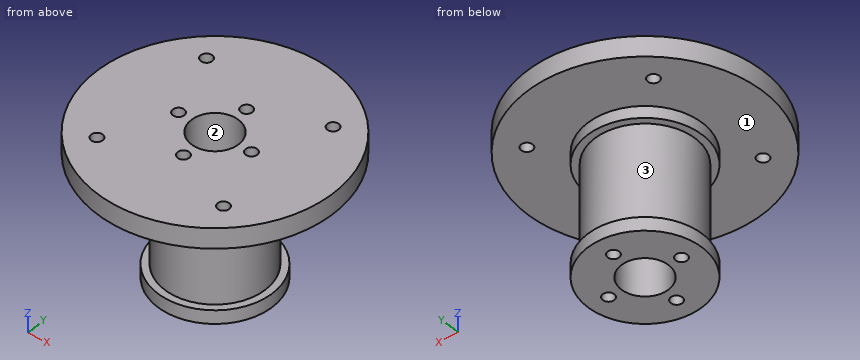
Solid Edge part; units mm, degrees
sketch "Sketch1" plane through (0, 0, 0) normal (0, 0, 1) x (1, 0, 0)
  circle A0 centre (0, 0) radius 17
  circle A1 centre (0, 0) radius 7
  circle A2 centre (11, 0) radius 1.7
  circle A3 centre (0, 11) radius 1.7
  circle A4 centre (-11, 0) radius 1.7
  circle A5 centre (0, -11) radius 1.7
extrude "Protrusion1" add sketch "Sketch1" along normal blind 4
sketch "Sketch2" plane through (0, 0, 4) normal (0, 0, 1) x (1, 0, 0)
  circle A0 centre (0, 0) radius 14.925
  circle A1 centre (0, 0) radius 7
  circle A2 centre (11, 0) radius 1.7
  circle A3 centre (0, 11) radius 1.7
  circle A4 centre (-11, 0) radius 1.7
  circle A5 centre (0, -11) radius 1.7
extrude "ExtrudedProtrusion_2" add sketch "Sketch2" along normal blind 29
sketch "Sketch3" plane through (0, 0, 33) normal (0, 0, 1) x (1, 0, 0)
  circle A0 centre (0, 0) radius 17
  circle A1 centre (0, 0) radius 7
  circle A2 centre (11, 0) radius 1.7
  circle A3 centre (0, 11) radius 1.7
  circle A4 centre (-11, 0) radius 1.7
  circle A5 centre (0, -11) radius 1.7
extrude "ExtrudedProtrusion_3" add sketch "Sketch3" along normal blind 3.5
sketch "Sketch4" plane through (0, 0, 36.5) normal (0, 0, 1) x (1, 0, 0)
  circle A0 centre (0, 0) radius 35
  circle A1 centre (0, 0) radius 7
  circle A2 centre (11, 0) radius 1.7
  circle A3 centre (0, 11) radius 1.7
  circle A4 centre (-11, 0) radius 1.7
  circle A5 centre (0, -11) radius 1.7
  circle A6 centre (19.0919, 19.0919) radius 1.7
  circle A7 centre (-19.0919, 19.0919) radius 1.7
  circle A8 centre (-19.0919, -19.0919) radius 1.7
  circle A9 centre (19.0919, -19.0919) radius 1.7
extrude "ExtrudedProtrusion_4" add sketch "Sketch4" along normal blind 6
Verification items for the finished model (mm, model axes). Face numbers are marked on the shaded views. Round coordinates to 2 decimals unless told otherwise and drop trailing zeros. Order: outer loops, then holes, each group sorted by start corner. A loop starts at its lowest first (then second) coordinate and runs counter-clockwise, first axis right, second up.
1) Depth check by flat-ended pin: pin 1 (5.5 mm diameter, centred on x = 11, y = 0, fed in from -Z); pin 2 (8 mm diameter, centred on y = -17, z = 37, fed in from -X); pin 3 (1.5 mm diameter, centred on x = 8, z = 12.5, fed in from +Y); pin 4 (4 mm diameter, centred on y = -13, z = 11, fed in from -X). Enter the tip coordinate at first touch or a pass-through.
Geometry says:
pin 1: stops at z = 0
pin 2: stops at x = -32.5
pin 3: stops at y = 13.05
pin 4: stops at x = -10.09
2) Draft check along X on the marked faces 1, 2 and 3. Enter one of: +X half, -X half, draft (parallel to the pull), parting line (faces both ways), or undercut.
Geometry says:
face 1: draft
face 2: undercut
face 3: parting line
3) Cross-section at B-B, the plane y = -3. Record the cut outline in (x, z), plus the area to 3 significant figures.
Geometry says:
outline: (-34.87, 36.5) - (-16.73, 36.5) - (-16.73, 33) - (-14.62, 33) - (-14.62, 4) - (-16.73, 4) - (-16.73, 0) - (-6.32, 0) - (-6.32, 42.5) - (-34.87, 42.5) - close; (6.32, 0) - (16.73, 0) - (16.73, 4) - (14.62, 4) - (14.62, 33) - (16.73, 33) - (16.73, 36.5) - (34.87, 36.5) - (34.87, 42.5) - (6.32, 42.5) - close
area: 980 mm2
4) Cross-section at C-C, the plane z = 39. Give the number of separate pieces and of enclosed holes in the cut face, plus the area to 3 significant figures.
Geometry says:
separate pieces: 1
enclosed holes: 9
area: 3,620 mm2
5) Cross-section at D-D, the plane x = -11. Record the cut outline in (y, z).
Geometry says:
outline: (-33.23, 36.5) - (-12.96, 36.5) - (-12.96, 33) - (-10.09, 33) - (-10.09, 4) - (-12.96, 4) - (-12.96, 0) - (-1.7, 0) - (-1.7, 42.5) - (-33.23, 42.5) - close; (1.7, 0) - (12.96, 0) - (12.96, 4) - (10.09, 4) - (10.09, 33) - (12.96, 33) - (12.96, 36.5) - (33.23, 36.5) - (33.23, 42.5) - (1.7, 42.5) - close
6) Material ranges on line 1 (Y direction, x = 0, z = 17.5) (3 decimals); line 2 (Z direction, x = -3.5, y = -23.5); line 3 (Y direction, x = 11, z = 37.5), recorded low to high.
Geometry says:
line 1: y = -14.925 to -12.7, -9.3 to -7, 7 to 9.3, 12.7 to 14.925
line 2: z = 36.5 to 42.5
line 3: y = -33.23 to -1.7, 1.7 to 33.23
7) Cross-section at A-A, the plane x = 0. Record the cut outline in (y, z) (3 decimals), plus the area to 3 significant figures.
Geometry says:
outline: (-35, 36.5) - (-17, 36.5) - (-17, 33) - (-14.925, 33) - (-14.925, 4) - (-17, 4) - (-17, 0) - (-12.7, 0) - (-12.7, 42.5) - (-35, 42.5) - close; (-9.3, 0) - (-7, 0) - (-7, 42.5) - (-9.3, 42.5) - close; (7, 0) - (9.3, 0) - (9.3, 42.5) - (7, 42.5) - close; (12.7, 0) - (17, 0) - (17, 4) - (14.925, 4) - (14.925, 33) - (17, 33) - (17, 36.5) - (35, 36.5) - (35, 42.5) - (12.7, 42.5) - close
area: 657 mm2
